```python
from build123d import *

# Parameters (mm, degrees)
EXTRUDE_1_DEPTH = 5
SKETCH_2_R      = 6.1
EXTRUDE_2_DEPTH = 13.8
SKETCH_3_W      = 0.639470974
SKETCH_3_H      = 3.15167837
SKETCH_3_W_2    = 0.411088483
SKETCH_3_H_2    = 2.90045763
EXTRUDE_3_DEPTH = 5.2


with BuildPart() as part:
    # 草图1 → 凸台-拉伸1 (new body)
    with BuildSketch(Plane.XY):
        Polygon((8, 0), (4, 6.92820323), (-4, 6.92820323), (-8, 0), (-4, -6.92820323), (4, -6.92820323), align=None)
    extrude(amount=EXTRUDE_1_DEPTH)

    # 草图2 → 凸台-拉伸2 (add)
    with BuildSketch(Plane(origin=(0, 0, 0), x_dir=(-1, 0, 0), z_dir=(0, 0, -1))):
        with Locations(Location((0, 0, 0), (0, 0, 180))):
            Circle(SKETCH_2_R)
    extrude(amount=EXTRUDE_2_DEPTH)

    # 草图3 → 凸台-拉伸3 (add)
    with BuildSketch(Plane(origin=(0, 0, -13.8), x_dir=(-1, 0, 0), z_dir=(0, 0, -1))):
        with Locations((-4.053789208, -0.308316362)):
            Rectangle(SKETCH_3_W, SKETCH_3_H)
        with Locations((4.213656952, -0.433926732)):
            Rectangle(SKETCH_3_W_2, SKETCH_3_H_2)
    extrude(amount=EXTRUDE_3_DEPTH)


solid = part.part
```
Model file for the job. Use its own axes, mm. A direction names the side the tool comes from. Round coordinates to 2 decimals unless told otherwise and drop trailing zeros. Order: outer loops, then holes, each group sorted by start corner. A loop starts at its lowest first (then second) coordinate and runs counter-clockwise, first axis right, second up. Notation, with made-up numbers: (6, -9) -> (48, -9) arc R16 ccw to (48, 11) -> close; hole circle Ø5 at (26.25, 66). An arc over 180 degrees is marked (long way). Use one line per item in the form item = value.
Item 1: Drill centre lines: line 1 (X direction, y = -0.5, z = -15.75); line 2 (Y direction, x = -0.25, z = -4.5); line 3 (Z direction, x = 5.75, y = 0.5). Where is each one in solid material? Low to high.
Returned:
line_1 = -4.42 to -4.01, 3.73 to 4.37
line_2 = -6.09 to 6.09
line_3 = -13.8 to 5
Item 2: Pull direction X, two halves, no side cores. Call faces 5 (the face through (0, 6.928, 2)), 6 (the face through (6.028, 3.416, 2.465)), 7 (the face through (3.734, 0, -16)), 8 (the face through (-6.094, -0.268, -6.803)): released by +X, released by -X, zero draft, split by the parting line, or undercut.
Returned:
face_5 = zero draft
face_6 = released by +X
face_7 = undercut
face_8 = split by the parting line
Item 3: Cut at D-D, the plane z = -10.25. Write the cut outline in (x, y).
Returned:
outline = circle Ø12.2 at (0, 0)
Item 4: Cut at B-B, the plane x = 0. Write the cut outline in (y, z).
Returned:
outline = (-6.93, 0) -> (-6.1, 0) -> (-6.1, -13.8) -> (6.1, -13.8) -> (6.1, 0) -> (6.93, 0) -> (6.93, 5) -> (-6.93, 5) -> close
Item 5: Flat gauge pins, fed straight in: pin 1 Ø1.6 at (y, z) = (-0.5, -16.5) entering from -X; pin 2 Ø0.9 at (y, z) = (-1, -16.5) entering from +X; pin 3 Ø6 at (y, z) = (-1.5, 1.5) entering from -X; pin 4 Ø1 at (x, y) = (3, -0.5) entering from -Z. Where does each tip first touch, or does it go through?
Returned:
pin_1 = -4.42
pin_2 = 4.37
pin_3 = -8
pin_4 = -13.8
Item 6: Cut at C-C, the plane y = -3.25. Write the cut outline in (x, z), and give its area (3 significant figures).
Returned:
outline = (-6.12, 0) -> (-5.16, 0) -> (-5.16, -13.8) -> (5.16, -13.8) -> (5.16, 0) -> (6.12, 0) -> (6.12, 5) -> (-6.12, 5) -> close
area = 204 mm^2
Item 7: Cut at A-A, the plane z = -15.5. Write the cut outline in (x, y), and give its area (3 significant figures).
Returned:
outline = (-4.42, -1.88) -> (-4.01, -1.88) -> (-4.01, 1.02) -> (-4.42, 1.02) -> close; (3.73, -1.88) -> (4.37, -1.88) -> (4.37, 1.27) -> (3.73, 1.27) -> close
area = 3.21 mm^2
Item 8: Tool access for faces 1 (the face through (-4.419, 0, -16)), 2 (the face through (6, 2, 0)), 3 (the face through (-4.008, 0, -16)), 4 (the face through (4.374, 0, -16)): list every direction of +Z, -Z, +X, -X, +Y, -Y with a clear straight run to the whole face (end or side of a thin tool).
Returned:
face_1 = -Z, -X, +Y, -Y
face_2 = -Z
face_3 = -Z, +Y, -Y
face_4 = -Z, +X, +Y, -Y
